Could you check a few things on this model? Use its own coordinates, in mm. Face numbers are marked on the shaded views. A direction names the side the tool comes from. Round coordinates to 2 decimals unless told otherwise and drop trailing zeros. Loops run counter-clockwise (first coordinate to the right, second up) from the corner with the lowest first, then second, coordinate; pieces in that order, holes last. Notation, with made-up numbers: (62, -33.75) -> (85, -33.75) arc R32 ccw to (85, 3.25) -> close; hole circle Ø9 at (46, -12). An arc over 180 degrees is marked (long way). One line per item, written item: value.
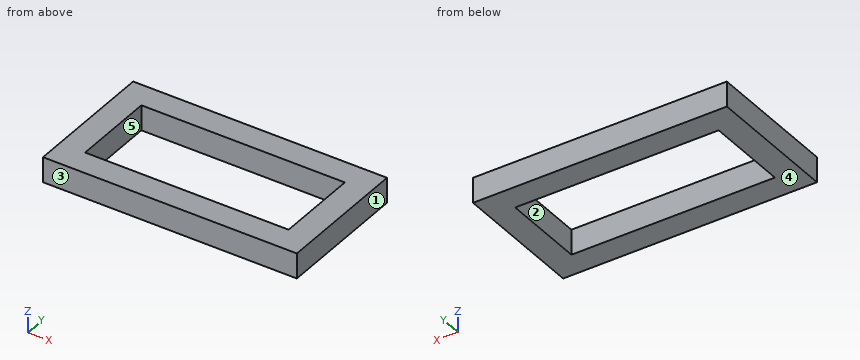
from build123d import *

# Parameters (mm, degrees)
SKETCH1_W           = 14.098000526
SKETCH1_H           = 7.448000431
SKETCH1_W_2         = 11.300000787
SKETCH1_H_2         = 4.650000215
BOSS_EXTRUDE1_DEPTH = 1.398000121


with BuildPart() as part:
    # Sketch1 → Boss-Extrude1 (new body)
    with BuildSketch(Plane.XY.offset(1.398000121)):
        with Locations((7.049000263, 3.724000216)):
            Rectangle(SKETCH1_W, SKETCH1_H)
        with Locations((7.048000515, 3.723000229)):
            Rectangle(SKETCH1_W_2, SKETCH1_H_2, mode=Mode.SUBTRACT)
    extrude(amount=-BOSS_EXTRUDE1_DEPTH)


solid = part.part
(1) If I drill on L1, parallel to Y at x = 6.25, z = 0.75; L2, parallel to X at y = 2.75, z = 0.2, over which ranges is the centre line in solid material (lowest first)?
Recorded:
L1: 0 to 1.4, 6.05 to 7.45
L2: 0 to 1.4, 12.7 to 14.1
(2) If we section it at A-A, the plane y = 2.25: Please give me the cut outline in (x, z), then the cut area to 3 significant figures.
Recorded:
outline: (0, 0) -> (1.4, 0) -> (1.4, 1.4) -> (0, 1.4) -> close; (12.7, 0) -> (14.1, 0) -> (14.1, 1.4) -> (12.7, 1.4) -> close
area: 3.91 mm²
(3) If we section it at B-B, the plane x = 4.75: Please give me the cut outline in (y, z), then the cut area to 3 significant figures.
Recorded:
outline: (0, 0) -> (1.4, 0) -> (1.4, 1.4) -> (0, 1.4) -> close; (6.05, 0) -> (7.45, 0) -> (7.45, 1.4) -> (6.05, 1.4) -> close
area: 3.91 mm²
(4) Thinking about a two-plate mould opening in Y: for the marked faces 3, 4 and 5, which applies, released by +Y, released by -Y, zero draft, split by the parting line, or undercut?
Recorded:
face 3: released by -Y
face 4: zero draft
face 5: undercut
(5) For the marked faces 1 and 2, which set-ups out of +Z, -Z, +X, -X, +Y, -Y let a thin tool reach every point of the face, with its end or its side?
Recorded:
face 1: +Z, -Z, +X, +Y, -Y
face 2: +Z, -Z
(6) If we section it at C-C, the plane z = 0.45: Please give me the cut outline in (x, y), then the cut area to 3 significant figures.
Recorded:
outline: (0, 0) -> (14.1, 0) -> (14.1, 7.45) -> (0, 7.45) -> close; hole (1.4, 1.4) -> (12.7, 1.4) -> (12.7, 6.05) -> (1.4, 6.05) -> close
area: 52.5 mm²
